Check sheet for the drawn part. Datum: minimum x, y, z corner. Units: mm. A direction names the side the tool comes from. Round coordinates to 2 decimals unless told otherwise and drop trailing zeros. Write each loop counter-clockwise with the first axis right and the second up, starting at its lowest first coordinate (ties: lowest second). Pieces come first, ordered by that corner, then holes. Notation, with made-up numbers: M 65.25,43 L 89.25,43 A27 cw 89.25,82 Z; hole C -7.75,89.5 d6. An arc over 180 degrees is marked long. Answer in a Markdown table with one row per item. Add a question column.
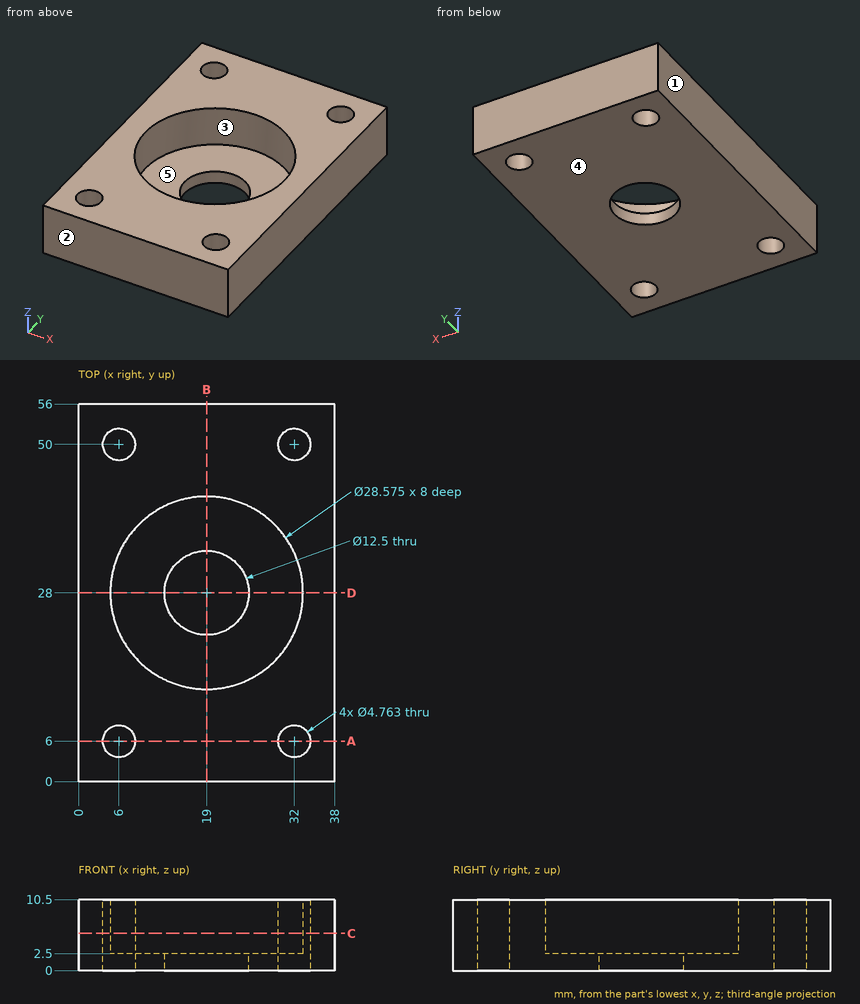
Item 1: Mould release check, pull along X, two halves, no side actions. Record for the marked faces 1, 2 and 3: +X half, -X half, draft (parallel to the pull), parting line (faces both ways), or undercut.
Item 2: Gauge pin test, flat ends, axial feed: pin 1 Ø4 at (x, y) = (32, 6) entering from +Z; pin 2 Ø14.5 at (x, y) = (20.5, 28.5) entering from +Z. Record the tip position at first contact, or that the pin passes through.
Item 3: Section check D-D, the plane y = 28. Record the boundary of the cut face in (x, z), and give its area (3 significant figures).
Item 4: Section check C-C, the plane z = 5.5. Record the boundary of the cut face in (x, y) (1 decimal), and give its area (3 significant figures).
Item 5: Section check A-A, the plane y = 6. Record the boundary of the cut face in (x, z).
Item 6: Section check B-B, the plane x = 19. Record the boundary of the cut face in (y, z).
Item 7: Scan lines: probe 1 along Y at (x, z) = (19.5, 4.25); probe 2 along Y at (x, z) = (32, 5.25) (1 decimal); probe 3 along Y at (x, z) = (30, 1.5) (1 decimal). Record each from-to range of solid material in increasing order. Write a range as from..to.
Item 8: Access from +Z, -Z, +X, -X, +Y, -Y to the whole of each face (thin tool, end or side, straight path). Record for the marked faces 4 and 5.
Result sheet:
| question | item | result |
|---|---|---|
| 1 | face 1 | -X half |
| 1 | face 2 | draft |
| 1 | face 3 | undercut |
| 2 | pin 1 | passes through |
| 2 | pin 2 | stops at z = 2.5 |
| 3 | outline | M 0,0 L 12.75,0 L 12.75,2.5 L 4.71,2.5 L 4.71,10.5 L 0,10.5 Z; M 25.25,0 L 38,0 L 38,10.5 L 33.29,10.5 L 33.29,2.5 L 25.25,2.5 Z |
| 3 | area | 139 mm^2 |
| 4 | outline | M 0,0 L 38,0 L 38,56 L 0,56 Z; hole C 6,6 d4.8; hole C 6,50 d4.8; hole C 19,28 d28.6; hole C 32,6 d4.8; hole C 32,50 d4.8 |
| 4 | area | 1,420 mm^2 |
| 5 | outline | M 0,0 L 3.62,0 L 3.62,10.5 L 0,10.5 Z; M 8.38,0 L 29.62,0 L 29.62,10.5 L 8.38,10.5 Z; M 34.38,0 L 38,0 L 38,10.5 L 34.38,10.5 Z |
| 6 | outline | M 0,0 L 21.75,0 L 21.75,2.5 L 13.71,2.5 L 13.71,10.5 L 0,10.5 Z; M 34.25,0 L 56,0 L 56,10.5 L 42.29,10.5 L 42.29,2.5 L 34.25,2.5 Z |
| 7 | probe 1 | y = 0..13.72, 42.28..56 |
| 7 | probe 2 | y = 0..3.6, 8.4..22.1, 33.9..47.6, 52.4..56 |
| 7 | probe 3 | y = 0..4.7, 7.3..48.7, 51.3..56 |
| 8 | face 4 | -Z, +X, -X, +Y, -Y |
| 8 | face 5 | +Z |
